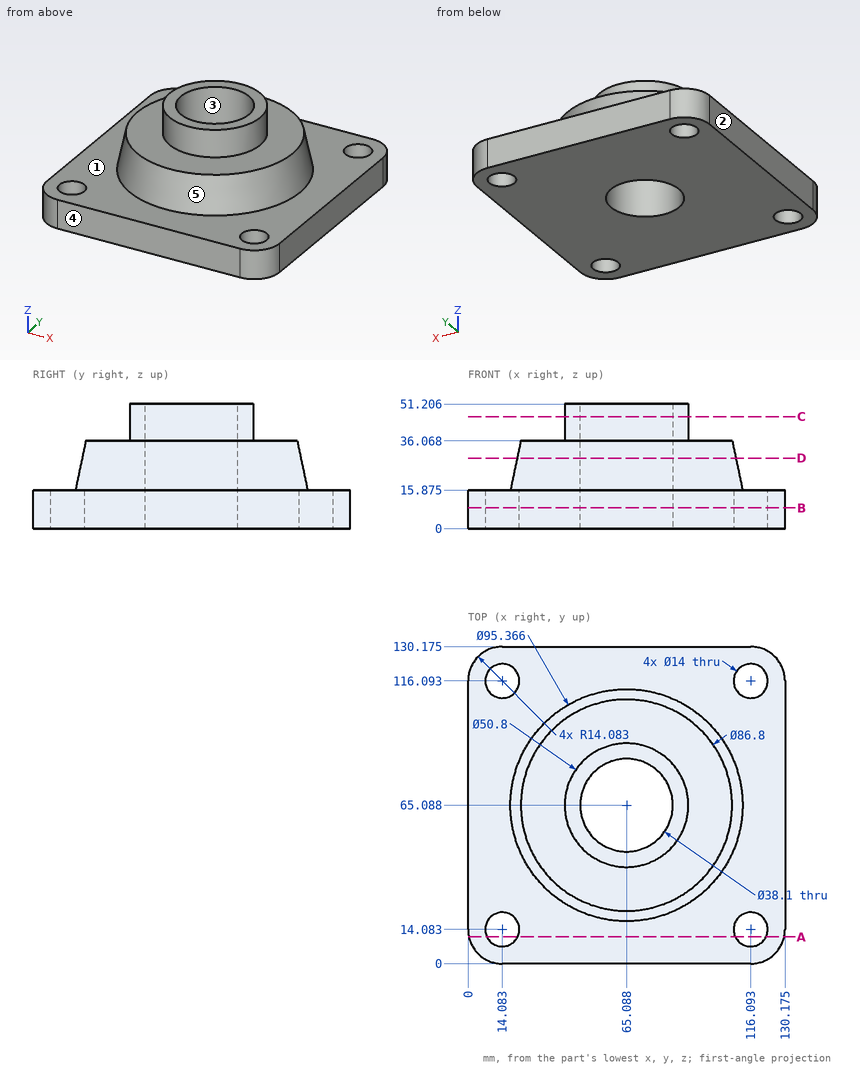
Part print with two shaded views. Sizes in mm from the minimum x, y, z corner. A direction names the side the tool comes from. Coordinates: 2 decimals unless noted, no trailing zeros. Order: outer loops, then holes, each group sorted by start corner. A loop starts at its lowest first (then second) coordinate and runs counter-clockwise, first axis right, second up. Notation, with made-up numbers: (-25.5, 85.25) - (17.5, 85.25) arc R27 cw to (17.5, 102.25) - close; hole circle Ø6 at (16.25, -36). An arc over 180 degrees is marked (long way). Write item = value, one per line. Start each with the question number.
1) Wall check: line 1 along Y through (x, z) = (18, 8) (1 decimal); line 2 along X through (y, z) = (60.5, 5.5) (1 decimal); line 3 along Y through (x, z) = (52, 5.5) (1 decimal). Give the ranges that are in metal, low to high. Write a range as from..to.
2) Saw through at D-D on z = 29. Write the cut outline in (x, y).
3) Saw through at A-A on y = 11. Write the cut outline in (x, z) (1 decimal).
4) Saw through at B-B on z = 8.5. Count the separate pieces of the cut face and the enclosed holes in it, then the cut area to 3 significant figures.
5) Two-plate mould, pull along X, no slides. Class the marked faces 3, 4 and 5: pulls with the +X half, pulls with the -X half, needs draft (parallel to the pull), parting line crosses it, or undercut.
6) Saw through at C-C on z = 46. Write the cut outline in (x, y).
7) 3-axis set-ups, long thin cutter, end or side, ignore diameter. For the marked faces 1 and 2: which of +Z, -Z, +X, -X, +Y, -Y reach the whole face in a straight line?
8) Flat gauge pins, fed straight in: pin 1 Ø3 at (x, z) = (71.5, 33.5) entering from +Y; pin 2 Ø8 at (y, z) = (59, 26) entering from -X; pin 3 Ø3 at (x, z) = (41, 42.5) entering from -Y. Where does each tip first touch, or does it go through?
From the geometry:
q1.line_1 = 0..8.3, 19.9..110.3, 121.9..130.2
q1.line_2 = 0..46.6, 83.6..130.2
q1.line_3 = 0..51.2, 78.9..130.2
q2.outline = circle Ø89.8 at (65.09, 65.09); hole circle Ø38.1 at (65.09, 65.09)
q3.outline = (0.3, 0) - (7.8, 0) - (7.8, 15.9) - (0.3, 15.9) - close; (20.4, 0) - (109.8, 0) - (109.8, 15.9) - (20.4, 15.9) - close; (122.4, 0) - (129.8, 0) - (129.8, 15.9) - (122.4, 15.9) - close
q4.separate_pieces = 1
q4.enclosed_holes = 5
q4.area = 15,000 mm^2
q5.face_3 = undercut
q5.face_4 = needs draft
q5.face_5 = parting line crosses it
q6.outline = circle Ø50.8 at (65.09, 65.09); hole circle Ø38.1 at (65.09, 65.09)
q7.face_1 = +Z
q7.face_2 = +Z, -Z, -X, +Y, -Y
q8.pin_1 = 108.94
q8.pin_2 = 18.99
q8.pin_3 = 53.47
